from build123d import *

# Parameters (mm, degrees)
BOSS_EXTRUDE1_DEPTH = 45
BOSS_EXTRUDE2_START = -10
BOSS_EXTRUDE2_DEPTH = 70
SKETCH5_R           = 25
SKETCH5_R_2         = 15
BOSS_EXTRUDE3_DEPTH = 30
RIB3_START          = -5
RIB3_DEPTH          = 10


with BuildPart() as part:
    # Sketch1 → Boss-Extrude1 (new, symmetric)
    with BuildSketch(Plane(origin=(0, 0, 0), x_dir=(0, 0, -1), z_dir=(1, 0, 0))):
        Polygon((-20.642857143, -6.642857143), (-30.642857143, -6.642857143), (-30.642857143, 8.357142857), (19.357142857, 8.357142857), (19.357142857, -6.642857143), (9.357142857, -6.642857143), (9.357142857, -1.642857143), (-20.642857143, -1.642857143), align=None)
    extrude(amount=BOSS_EXTRUDE1_DEPTH, both=True)

    # Sketch2 → Boss-Extrude2 (add)
    with BuildSketch(Plane(origin=(45, 0, 0), x_dir=(0, 0, -1), z_dir=(1, 0, 0)).offset(BOSS_EXTRUDE2_START)):
        with BuildLine():
            Line((19.357142857, 8.357142857), (19.357142857, 38.357142857))
            ThreePointArc((19.357142857, 38.357142857), (20.821608951, 41.892676763), (24.357142857, 43.357142857))
            Line((24.357142857, 43.357142857), (94.357142857, 43.357142857))
            ThreePointArc((94.357142857, 43.357142857), (97.892676763, 41.892676763), (99.357142857, 38.357142857))
            Line((99.357142857, 38.357142857), (99.357142857, 8.357142857))
            Line((99.357142857, 8.357142857), (109.357142857, 8.357142857))
            Line((109.357142857, 8.357142857), (109.357142857, 38.357142857))
            ThreePointArc((109.357142857, 38.357142857), (104.963744575, 48.963744575), (94.357142857, 53.357142857))
            Line((94.357142857, 53.357142857), (24.357142857, 53.357142857))
            ThreePointArc((24.357142857, 53.357142857), (13.750541139, 48.963744575), (9.357142857, 38.357142857))
            Line((9.357142857, 38.357142857), (9.357142857, 8.357142857))
            Line((9.357142857, 8.357142857), (19.357142857, 8.357142857))
        make_face()
    extrude(amount=-BOSS_EXTRUDE2_DEPTH)

    # Sketch5 → Boss-Extrude3 (add)
    with BuildSketch(Plane(origin=(0, 53.357142857, 0), x_dir=(1, 0, 0), z_dir=(0, 1, 0))):
        with Locations(Location((0, 59.357142857, 0), (0, 0, 270))):
            Circle(SKETCH5_R)
        with Locations(Location((0, 59.357142857, 0), (0, 0, 270))):
            Circle(SKETCH5_R_2, mode=Mode.SUBTRACT)
    extrude(amount=BOSS_EXTRUDE3_DEPTH)

    # Rib3: read off the stored shape, not the designer's step
    # Rib3 outline → Rib3 (add)
    with BuildSketch(Plane(origin=(0, 0, 0), x_dir=(0, 0, -1), z_dir=(1, 0, 0)).offset(RIB3_START)):
        with BuildLine():
            Line((34.862245429, 83.357142857), (34.357142857, 83.357142857))
            Line((34.357142857, 83.357142857), (-30.642857143, 8.357142857))
            Line((-30.642857143, 8.357142857), (9.357142857, 8.357142857))
            Line((9.357142857, 8.357142857), (9.357142857, 38.357142857))
            ThreePointArc((9.357142857, 38.357142857), (13.750541139, 48.963744575), (24.357142857, 53.357142857))
            Line((24.357142857, 53.357142857), (34.862245429, 53.357142857))
            Line((34.862245429, 53.357142857), (34.862245429, 83.357142857))
        make_face()
    extrude(amount=RIB3_DEPTH)


solid = part.part
Work out the finished part from the listing and answer in its coordinate system (mm). A direction names the side the tool comes from. Coordinates: 2 decimals unless noted, no trailing zeros. Loops run counter-clockwise (first coordinate to the right, second up) from the corner with the lowest first, then second, coordinate; pieces in that order, holes last. Notation, with made-up numbers: (-32.5, -31.5) -> (-20.5, -31.5) arc R20 cw to (-20.5, 4.5) -> close; hole circle Ø10 at (61, -9.5). An arc over 180 degrees is marked (long way). Write each question's results on one line, items separated by ' | '. Start each with the question number.
1) Find section A-A on y = 20. Determine the outline of the cut face in (x, z).
2) Find section D-D on y = 56.5. Determine the outline of the cut face in (x, z), then the cut area to 3 significant figures.
3) Find section B-B on x = -27. Determine the outline of the cut face in (y, z), then the cut area to 3 significant figures.
4) The mould has two halves that part along X. Classify faces 1 (the cylindrical face through (1.029, 68.147, -84.336)), 2 (the flat face through (-10.8, 83.357, -48.6)), 3 (the cylindrical face through (0.66, 68.147, -74.343)), 4 (the flat face through (-35, 46, -59)): pulls with the +X half, pulls with the -X half, needs draft (parallel to the pull), parting line crosses it, or undercut.
5) Flat-ended cylindrical pins translate along their axes: P1, Ø5, axis at x = -28.5, z = -70, coming from the -Y side; P2, Ø22.5, axis at y = 36.5, z = -45.5, coming from the +X side; P3, Ø5, axis at x = -14, z = -103.5, coming from the -Y side; P4, Ø22.5, axis at y = 25.5, z = -47, coming from the -X side. Find the tip coordinate at first contact, or state that the pin passes through.
6) For faces 5 (the cylindrical face through (-19.79, 49.08, -13.87)), 6 (the cylindrical face through (20.21, 49.08, -13.87)), 7 (the flat face through (1, -1.643, 5)), determine the directions among +Z, -Z, +X, -X, +Y, -Y from which every point of the face is accessible in a straight line to the end or side of a thin tool.
7) Consider line 1 along Z through (x, y) = (32, -3); line 2 along Z through (x, y) = (-22, 32.5); line 3 along Y through (x, z) = (-20, 17). Determine where each line is inside the solid, lowest interval first.
8) Find section C-C on z = -4. Determine the outline of the cut face in (x, y), then the cut area to 3 significant figures.
Response values:
1) outline: (-35, -109.36) -> (35, -109.36) -> (35, -99.36) -> (-35, -99.36) -> close; (-35, -19.36) -> (35, -19.36) -> (35, -9.36) -> (5, -9.36) -> (5, 20.55) -> (-5, 20.55) -> (-5, -9.36) -> (-35, -9.36) -> close
2) outline: (-5, -34.86) arc R25 ccw (long way) to (5, -34.86) -> (5, -11.08) -> (-5, -11.08) -> close; hole circle Ø30 at (0, -59.36) | area: 1,490 mm^2
3) outline: (-6.64, -19.36) -> (38.36, -19.36) arc R5 cw to (43.36, -24.36) -> (43.36, -94.36) arc R5 cw to (38.36, -99.36) -> (8.36, -99.36) -> (8.36, -109.36) -> (38.36, -109.36) arc R15 ccw to (53.36, -94.36) -> (53.36, -24.36) arc R15 ccw to (38.36, -9.36) -> (8.36, -9.36) -> (8.36, 30.64) -> (-6.64, 30.64) -> (-6.64, 20.64) -> (-1.64, 20.64) -> (-1.64, -9.36) -> (-6.64, -9.36) -> close | area: 2,210 mm^2
4) face 1: parting line crosses it | face 2: needs draft | face 3: undercut | face 4: pulls with the -X half
5) P1: stops at y = 43.36 | P2: stops at x = 35 | P3: stops at y = 8.36 | P4: passes through
6) face 5: +Z, -X, +Y | face 6: +Z, +X, +Y | face 7: +X, -X, -Y
7) line 1: z = -19.36 to -9.36, 20.64 to 30.64 | line 2: z = -109.36 to -99.36, -19.36 to -9.36 | line 3: y = -1.64 to 8.36
8) outline: (-45, -1.64) -> (45, -1.64) -> (45, 8.36) -> (5, 8.36) -> (5, 48.33) -> (-5, 48.33) -> (-5, 8.36) -> (-45, 8.36) -> close | area: 1,300 mm^2
